from build123d import *

# Parameters (mm, degrees)
F1_DEPTH = 63.5
F2_DEPTH = 25.4
F3_DEPTH = 7.9375
F5_R     = 6.35


with BuildPart() as f1:
    # F0 (on Front) → F1 (new body, symmetric)
    with BuildSketch(Plane.XZ):
        Polygon((-41.275, 9.525), (-41.275, -9.525), (41.275, -9.525), (41.275, 9.525), (22.225, 9.525), align=None)
    extrude(amount=F1_DEPTH, both=True)

    # F0 (on Front) → F2 (join, symmetric)
    with BuildSketch(Plane.XZ):
        with BuildLine():
            Line((22.225, 9.525), (41.275, 9.525))
            Line((41.275, 9.525), (41.275, 27.0002))
            ThreePointArc((41.275, 27.0002), (45.92468, 38.22552), (57.15, 42.8752))
            Line((57.15, 42.8752), (60.325, 42.8752))
            Line((60.325, 42.8752), (60.325, 61.9252))
            Line((60.325, 61.9252), (57.15, 61.9252))
            ThreePointArc((57.15, 61.9252), (32.454296, 51.695904), (22.225, 27.0002))
            Line((22.225, 27.0002), (22.225, 9.525))
        make_face()
    extrude(amount=F2_DEPTH, both=True)

    # F0 (on Front) → F3 (join, symmetric)
    with BuildSketch(Plane.XZ):
        with BuildLine():
            add(Edge.make_bspline(
                [(-41.275, 9.525), (-31.276178, 51.95152), (19.80542, 62.86972), (57.15, 61.9252)],
                knots=[0, 0, 0, 0, 111.504536, 111.504536, 111.504536, 111.504536], degree=3))
            Line((-41.275, 9.525), (22.225, 9.525))
            Line((22.225, 9.525), (22.225, 27.0002))
            ThreePointArc((22.225, 27.0002), (32.454296, 51.695904), (57.15, 61.9252))
        make_face()
    extrude(amount=F3_DEPTH, both=True)

    # F0 (on Front) → F4 (revolve)
    with BuildSketch(Plane.XZ):
        Polygon((82.134529, 66.675), (82.134529, 61.9252), (82.134529, 42.8752), (82.134529, 38.1), (111.125, 38.1), (111.125, 66.675), align=None)
    revolve(axis=Axis((82.134529, 0, 52.3875), (0, 0, -1)))

    # F5
    f5_edges = [f1.edges().sort_by_distance(p)[0] for p in [
        (41.275, -63.5, 0),
        (-41.275, -63.5, 0),
        (41.275, 63.5, 0),
        (-41.275, 63.5, 0),
    ]]
    fillet(f5_edges, radius=F5_R)


solid = f1.part
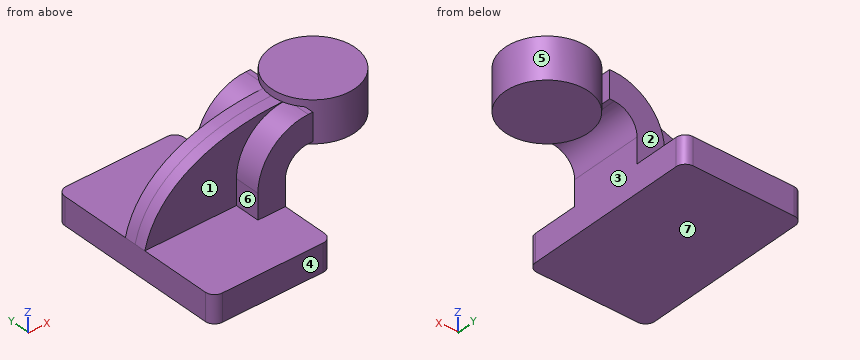
Work out the finished part from the listing and answer in its coordinate system (mm). Face numbers are marked on the shaded views. A direction names the side the tool comes from. Coordinates: 2 decimals unless noted, no trailing zeros. Loops run counter-clockwise (first coordinate to the right, second up) from the corner with the lowest first, then second, coordinate; pieces in that order, holes last. Notation, with made-up numbers: (26, -40) -> (49, -40) arc R23 cw to (49, -23) -> close; hole circle Ø5 at (15, 67.5). An arc over 180 degrees is marked (long way). Write each question's results on one line, items separated by ' | '. Start each with the question number.
1) Consider line 1 along Z through (x, y) = (5, 28) (3 decimals); line 2 along Y through (x, z) = (34.5, 48); line 3 along Y through (x, z) = (-15.5, 42.5). Determine where each line is inside the solid, lowest interval first.
2) For the marked faces 1, 2, 3 and 4, determine the directions among +Z, -Z, +X, -X, +Y, -Y from which every point of the face is accessible in a straight line to the end or side of a thin tool.
3) The mould has two halves that part along X. Classify the marked faces 5, 6 and 7: pulls with the +X half, pulls with the -X half, needs draft (parallel to the pull), parting line crosses it, or undercut.
4) Find section B-B on x = 93.5. Determine the outline of the cut face in (y, z) (3 decimals), then the cut area to 3 significant figures.
5) Flat-ended cylindrical pins translate along their axes: P1, Ø8, axis at x = -21.5, y = -15.5, coming from the +Z side (3 decimals); P2, Ø12, axis at x = 26, z = 52, coming from the -Y side; P3, Ø5, axis at y = 20, z = 16, coming from the -X side (3 decimals). Find the tip coordinate at first contact, or state that the pin passes through.
6) Find section A-A on y = 34. Determine the outline of the cut face in (x, z) (3 decimals).
Response values:
1) line 1: z = -9.525 to 9.525 | line 2: y = -25.4 to 25.4 | line 3: y = -7.94 to 7.94
2) face 1: +Z, -X, -Y | face 2: +Z, -X, +Y | face 3: -Z, +X, +Y, -Y | face 4: +Z, -Z, +X, -X, -Y
3) face 5: undercut | face 6: pulls with the -X half | face 7: needs draft
4) outline: (-26.67, 38.1) -> (26.67, 38.1) -> (26.67, 66.675) -> (-26.67, 66.675) -> close | area: 1,520 mm^2
5) P1: stops at z = 9.525 | P2: stops at y = -25.4 | P3: stops at x = 22.225
6) outline: (-41.275, -9.525) -> (41.275, -9.525) -> (41.275, 9.525) -> (-41.275, 9.525) -> close
